```python
from build123d import *

# Parameters (mm, degrees)
SKETCH1_W           = 24
SKETCH1_H           = 10.7
BOSS_EXTRUDE1_DEPTH = 1.5
SKETCH2_W           = 24
SKETCH2_H           = 2.4
BOSS_EXTRUDE2_DEPTH = 1.4
BOSS_EXTRUDE2_DRAFT = -10
FILLET1_R           = 1.5


with BuildPart() as part:
    # Sketch1 → Boss-Extrude1 (new body)
    with BuildSketch(Plane.XY):
        Rectangle(SKETCH1_W, SKETCH1_H)
    extrude(amount=BOSS_EXTRUDE1_DEPTH)


with BuildPart() as boss_extrude2_tool:
    # Sketch2 → Boss-Extrude2 (with draft: the straight prism first)
    with BuildSketch(Plane(origin=(0, 0, 0), x_dir=(-1, 0, 0), z_dir=(0, 0, -1))):
        Rectangle(SKETCH2_W, SKETCH2_H)
    extrude(amount=BOSS_EXTRUDE2_DEPTH)
    # Boss-Extrude2: the draft: its side faces are tilted about the plane it starts from
    boss_extrude2_sides = [boss_extrude2_tool.faces().sort_by_distance(p)[0] for p in [
        (12, 0, -0.7),
        (0, -1.2, -0.7),
        (-12, 0, -0.7),
        (0, 1.2, -0.7),
    ]]
    draft(boss_extrude2_sides, Plane(origin=(0, 0, 0), x_dir=(-1, 0, 0), z_dir=(0, 0, -1)), BOSS_EXTRUDE2_DRAFT)


with BuildPart() as part_1:
    add(part.part)

    # Boss-Extrude2: add boss_extrude2_tool
    add(boss_extrude2_tool.part)

    # Fillet1
    fillet1_edges = [part_1.edges().sort_by_distance(p)[0] for p in [
        (0, -5.35, 1.5),
        (-12, 0, 1.5),
        (0, 5.35, 1.5),
        (12, 0, 1.5),
    ]]
    fillet(fillet1_edges, radius=FILLET1_R - 0.0001)  # a hair under: the kernel refuses the full size


solid = part_1.part
```
Read the model definition and answer for the solid it produces. Units are mm, in the model's axes. A direction names the side the tool comes from. Coordinates: 2 decimals unless noted, no trailing zeros. Loops run counter-clockwise (first coordinate to the right, second up) from the corner with the lowest first, then second, coordinate; pieces in that order, holes last. Notation, with made-up numbers: (67, -37) - (85, -37) arc R25 cw to (85, -7) - close; hole circle Ø9 at (-30.75, 41.25). An arc over 180 degrees is marked (long way). Answer in a Markdown table with one row per item.
1. Straight lines are drawn through the part: line 1 (Z direction, x = -0.75, y = -2.75); line 2 (Y direction, x = -9.5, z = 0.85); line 3 (X direction, y = -0.25, z = -1.15). For each, find the intervals that lie inside material, in ascending order.
Conclusion:
| item | result |
|---|---|
| line 1 | z = 0 to 1.5 |
| line 2 | y = -5.09 to 5.09 |
| line 3 | x = -12.2 to 12.2 |
2. Given pin 1 (1.2 mm diameter, centred on x = -5.5, y = -3, fed in from -Z), flat-ended and moving along its own axis, determine where the tip first touches the part or whether it passes through.
Conclusion:
| item | result |
|---|---|
| pin 1 | stops at z = 0 |
3. Find section D-D, the plane z = 0.4. Write down the section's boundary in (x, y).
Conclusion:
| item | result |
|---|---|
| outline | (-11.95, -5.3) - (11.95, -5.3) - (11.95, 5.3) - (-11.95, 5.3) - close |
4. Which of the six approach directions +Z, -Z, +X, -X, +Y, -Y give full straight-line access (tool end or side, diameter ignored) to faces 1 (the face through (0, 0, -1.4)), 2 (the face through (0.17, -1.32, -0.69)), 3 (the face through (0.17, 1.32, -0.69))?
Conclusion:
| item | result |
|---|---|
| face 1 | -Z, +X, -X, +Y, -Y |
| face 2 | +X, -X, -Y |
| face 3 | +X, -X, +Y |
